The drawing under review shows one solid part. Ordinate dimensions are in mm from its lowest x, y, z. Coordinates: 2 decimals unless noted, no trailing zeros. Write each loop counter-clockwise with the first axis right and the second up, starting at its lowest first coordinate (ties: lowest second). Pieces come first, ordered by that corner, then holes. Notation, with made-up numbers: (-0.5, 24) - (5.5, 24) arc R16 ccw to (5.5, 35) - close; hole circle Ø5 at (-32.75, 77.25). An arc over 180 degrees is marked (long way). Use a Markdown table: item, result.
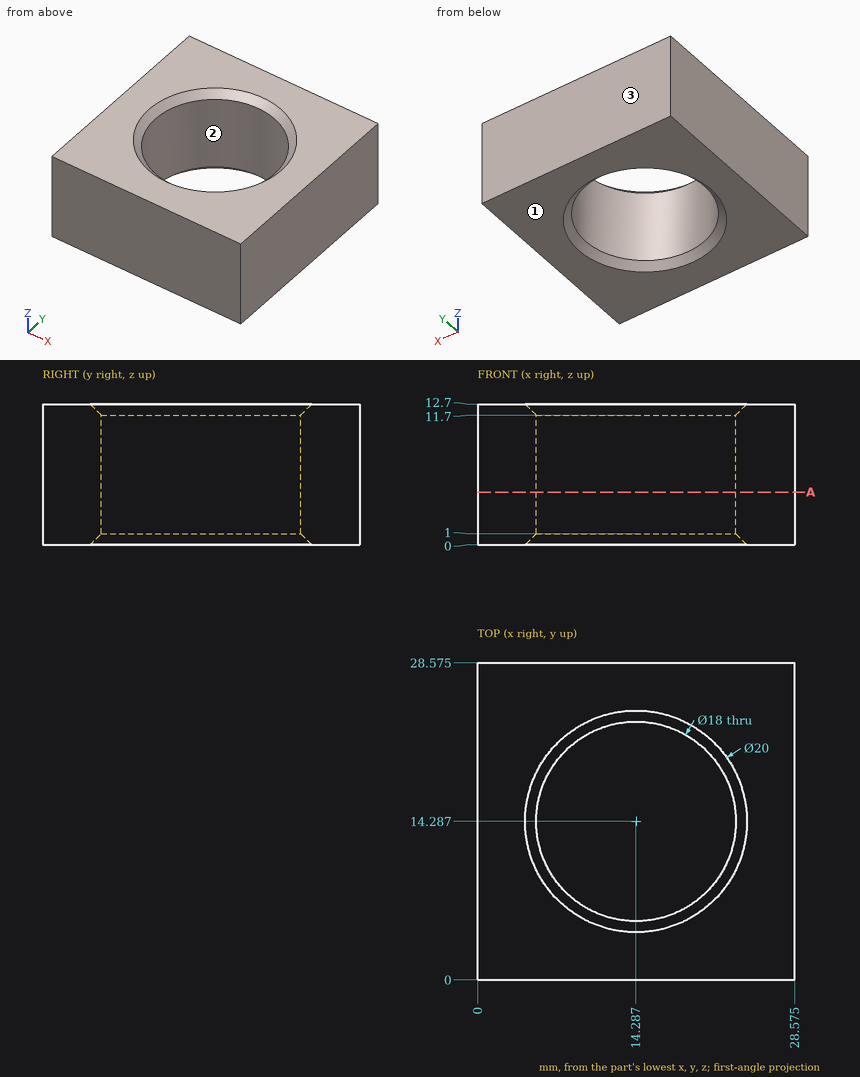
(1) Take a section at A-A on z = 4.75. Write out the cut boundary in (x, y) (1 decimal).
Determined:
| item | result |
|---|---|
| outline | (0, 0) - (28.6, 0) - (28.6, 28.6) - (0, 28.6) - close; hole circle Ø18 at (14.3, 14.3) |
(2) Draft analysis for pull direction Y (two halves, no side actions). For the marked faces 1, 2 and 3, state which applies: +Y half, -Y half, draft (parallel to the pull), parting line (faces both ways), or undercut.
Determined:
| item | result |
|---|---|
| face 1 | draft |
| face 2 | undercut |
| face 3 | +Y half |
(3) For pin 1 (5 mm diameter, centred on y = 3.5, z = 9.5, fed in from -X); pin 2 (3 mm diameter, centred on x = 20, y = 20, fed in from -Z), all flat-tipped, find the tip position at first contact; note any pin that passes through.
Determined:
| item | result |
|---|---|
| pin 1 | x = 0 |
| pin 2 | z = 0.42 |
(4) For L1, parallel to Y at x = 14.25, z = 2.75 (1 decimal); L2, parallel to Y at x = 17, z = 11.25 (1 decimal), list the stretches that pass through material, from the lowest coordinate up. Write a range as from..to.
Determined:
| item | result |
|---|---|
| L1 | 0..5.3, 23.3..28.6 |
| L2 | 0..5.7, 22.9..28.6 |
